```python
from build123d import *

# Parameters (mm, degrees)
F0_R     = 6.35
F0_R_2   = 9.017
F0_R_3   = 1.75
F1_DEPTH = 68.072
F2_DEPTH = 6.35
F3_DEPTH = 1.524
F4_DEPTH = 12.7
F5_R     = 0.2539
F6_SIZE  = 0.254
F7_R     = 3.81
F8_DEPTH = 2.286
F9_R     = 1.905


# Not quite as in the source:
# - a fillet or chamfer is up to 0.001 mm smaller than in the source, because OpenCascade refuses the exact size


with BuildPart() as f1:
    # F0 (on Front) → F1 (new body)
    with BuildSketch(Plane.XZ):
        with BuildLine():
            Line((-20.701, -10.541), (15.494, -10.541))
            ThreePointArc((15.494, -10.541), (4.953, 0), (15.494, 10.541))
            Line((15.494, 10.541), (-20.701, 10.541))
            ThreePointArc((-20.701, 10.541), (-23.3950768363, 9.4250768363), (-24.511, 6.731))
            Line((-24.511, 6.731), (-24.511, -6.731))
            ThreePointArc((-24.511, -6.731), (-23.3950768363, -9.4250768363), (-20.701, -10.541))
        make_face()
        with Locations((-13.335, -2.921)):
            Circle(F0_R, mode=Mode.SUBTRACT)
        with BuildLine():
            Line((15.494, -10.541), (20.701, -10.541))
            ThreePointArc((20.701, -10.541), (23.3950768363, -9.4250768363), (24.511, -6.731))
            Line((24.511, -6.731), (24.511, 0))
            Line((24.511, 0), (24.511, 6.731))
            ThreePointArc((24.511, 6.731), (23.3950768363, 9.4250768363), (20.701, 10.541))
            Line((20.701, 10.541), (15.494, 10.541))
            ThreePointArc((15.494, 10.541), (4.953, 0), (15.494, -10.541))
        make_face()
        with Locations((15.494, 0)):
            Circle(F0_R_2, mode=Mode.SUBTRACT)
        with Locations((15.494, 0)):
            Circle(F0_R_2)
        with Locations((-13.335, -2.921)):
            Circle(F0_R)
        with Locations((-13.335, -2.921)):
            Circle(F0_R_3, mode=Mode.SUBTRACT)
        with Locations((-13.335, -2.921)):
            Circle(F0_R_3)
    extrude(amount=-F1_DEPTH)

    # F0 (on Front) → F2 (join)
    with BuildSketch(Plane.XZ):
        with Locations((15.494, 0)):
            Circle(F0_R_2)
    extrude(amount=F2_DEPTH)

    # F0 (on Front) → F3 (join)
    with BuildSketch(Plane.XZ):
        with BuildLine():
            Line((-20.701, -10.541), (15.494, -10.541))
            ThreePointArc((15.494, -10.541), (4.953, 0), (15.494, 10.541))
            Line((15.494, 10.541), (-20.701, 10.541))
            ThreePointArc((-20.701, 10.541), (-23.3950768363, 9.4250768363), (-24.511, 6.731))
            Line((-24.511, 6.731), (-24.511, -6.731))
            ThreePointArc((-24.511, -6.731), (-23.3950768363, -9.4250768363), (-20.701, -10.541))
        make_face()
        with Locations((-13.335, -2.921)):
            Circle(F0_R, mode=Mode.SUBTRACT)
    extrude(amount=F3_DEPTH)

    # F0 (on Front) → F4 (cut)
    with BuildSketch(Plane.XZ):
        with Locations((-13.335, -2.921)):
            Circle(F0_R_3)
    extrude(amount=-F4_DEPTH, mode=Mode.SUBTRACT)

    # F5 (radius 0.254 in the source; OpenCascade refuses exactly that, so slightly less here)
    f5_edges = [f1.edges().sort_by_distance(p)[0] for p in [
        (15.494, -0.762, 10.541),
        (15.494, -0.762, -10.541),
    ]]
    fillet(f5_edges, radius=F5_R)

    # F6
    f6_edges = [f1.edges().sort_by_distance(p)[0] for p in [
        (6.477, -6.35, 0),
        (-19.685, -1.524, -2.921),
    ]]
    chamfer(f6_edges, length=F6_SIZE)

    # F7 (on face) → F8 (join)
    with BuildSketch(Plane(origin=(0, 0, -10.541), x_dir=(1, 0, 0), z_dir=(0, 0, -1))):
        with Locations((-14.605, -7.366)):
            Circle(F7_R)
        with Locations((14.605, -7.366)):
            Circle(F7_R)
        with Locations((-14.605, -60.706)):
            Circle(F7_R)
        with Locations((14.605, -59.182)):
            Circle(F7_R)
    extrude(amount=F8_DEPTH)

    # F9
    f9_edges = [f1.edges().sort_by_distance(p)[0] for p in [
        (-18.415, 7.366, -12.827),
        (10.795, 7.366, -12.827),
        (10.795, 59.182, -12.827),
        (-18.415, 60.706, -12.827),
    ]]
    fillet(f9_edges, radius=F9_R)


solid = f1.part
```
The model under review builds one solid part; all positions refer to its coordinate system, in mm. A direction names the side the tool comes from. Coordinates: 2 decimals unless noted, no trailing zeros. Write each loop counter-clockwise with the first axis right and the second up, starting at its lowest first coordinate (ties: lowest second). Pieces come first, ordered by that corner, then holes.
1) We need section A-A on y = 42.5. State the section outline as (x, z) points.
2) Machinability: for faces 5 (the face through (-11.666, 6.261, -2.395)), 6 (the face through (-23.37, 33.76, 9.45)), 7 (the face through (0, 34, -10.541)), which of the approach directions +Z, -Z, +X, -X, +Y, -Y give a long, thin tool a straight path to every point of the face, cutting with its end or side? Answer none if there is none.
3) To check wall thickness, follow probe 1 along Z at (x, y) = (18, 21.5); probe 2 along Y at (x, z) = (3, -6.5); probe 3 along Y at (x, z) = (-14, -10.75). State the ranges of each line that lie inside material, in increasing order.
4) We need section B-B on x = -1. State the section outline as (y, z) points.
5) The part is to be moulded in two halves that separate along Y. For faces 1 (the face through (13, 0, -9)), 2 (the face through (18.24, 6.22, -10.73)), 3 (the face through (0, 68.072, 0)), 4 (the face through (23.42, 33.56, 9.4)), say which applies: pulls with the +Y half, pulls with the -Y half, needs draft (parallel to the pull), parting line crosses it, or undercut.
6) Clearance check with flat-ended pins moving along their axes: pin 1 Ø3 at (x, z) = (-14, -2.5) entering from -Y; pin 2 Ø8 at (x, y) = (-3, 1) entering from -Z; pin 3 Ø10 at (x, z) = (-15, -2) entering from -Y. State where each tip first meets the part, or that it passes through.
Answer list:
1. outline: (-24.51, -6.73) arc R3.81 ccw to (-20.7, -10.54) - (20.7, -10.54) arc R3.81 ccw to (24.51, -6.73) - (24.51, 6.73) arc R3.81 ccw to (20.7, 10.54) - (-20.7, 10.54) arc R3.81 ccw to (-24.51, 6.73) - close
2. face 5: -Y
2. face 6: +Z, -X, +Y, -Y
2. face 7: -Z
3. probe 1: z = -10.54 to 10.54
3. probe 2: y = -1.52 to 68.07
3. probe 3: y = 3.6 to 11.13, 56.94 to 64.47
4. outline: (-1.52, -10.54) - (68.07, -10.54) - (68.07, 10.54) - (-1.52, 10.54) - close
5. face 1: pulls with the -Y half
5. face 2: undercut
5. face 3: pulls with the +Y half
5. face 4: needs draft
6. pin 1: stops at y = 0
6. pin 2: stops at z = -10.54
6. pin 3: stops at y = -1.52
